```python
from build123d import *

# Parameters (mm, degrees)
ESQUISSE1_W             = 140
ESQUISSE1_H             = 40
ESQUISSE1_R             = 2.75
ESQUISSE1_R_2           = 1.6
ESQUISSE1_R_3           = 12.5
BOSS_EXTRU_1_DEPTH      = 2
ENL_V_MAT_EXTRU_1_REACH = 4
CONG_1_R                = 2


with BuildPart() as part:
    # Esquisse1 → Boss.-Extru.1 (new body)
    with BuildSketch(Plane(origin=(0, 0, 0), x_dir=(1, 0, 0), z_dir=(0, 1, 0))):
        Rectangle(ESQUISSE1_W, ESQUISSE1_H)
        with Locations((-61, 0)):
            Circle(ESQUISSE1_R, mode=Mode.SUBTRACT)
        with Locations((-29, 0)):
            Circle(ESQUISSE1_R, mode=Mode.SUBTRACT)
        with Locations((29, 0)):
            Circle(ESQUISSE1_R, mode=Mode.SUBTRACT)
        with Locations((61, 0)):
            Circle(ESQUISSE1_R, mode=Mode.SUBTRACT)
        with Locations((-15.5, 15.5)):
            Circle(ESQUISSE1_R_2, mode=Mode.SUBTRACT)
        with Locations((15.5, 15.5)):
            Circle(ESQUISSE1_R_2, mode=Mode.SUBTRACT)
        with Locations((15.5, -15.5)):
            Circle(ESQUISSE1_R_2, mode=Mode.SUBTRACT)
        with Locations((-15.5, -15.5)):
            Circle(ESQUISSE1_R_2, mode=Mode.SUBTRACT)
        Circle(ESQUISSE1_R_3, mode=Mode.SUBTRACT)
    extrude(amount=BOSS_EXTRU_1_DEPTH)

    # Esquisse2 → Enlèv. mat.-Extru.1 (cut, up to next)
    with BuildSketch(Plane.XZ, mode=Mode.PRIVATE) as enl_v_mat_extru_1_sk1:
        Polygon((22, -20), (22, -7.5), (67, -7.5), (67, 7.5), (22, 7.5), (22, 20), (70, 20), (70, -20), align=None)
    enl_v_mat_extru_1_tool1 = extrude(enl_v_mat_extru_1_sk1.sketch, amount=-ENL_V_MAT_EXTRU_1_REACH, mode=Mode.PRIVATE) & part.part
    add(enl_v_mat_extru_1_tool1.solids().sort_by_distance((22.62482, 0, -13.75))[0], mode=Mode.SUBTRACT)
    # Esquisse2 → Enlèv. mat.-Extru.1 (cut, up to next)
    with BuildSketch(Plane.XZ, mode=Mode.PRIVATE) as enl_v_mat_extru_1_sk2:
        Polygon((-70, 20), (-70, -20), (-22, -20), (-22, -7.5), (-67, -7.5), (-67, 7.5), (-22, 7.5), (-22, 20), align=None)
    enl_v_mat_extru_1_tool2 = extrude(enl_v_mat_extru_1_sk2.sketch, amount=-ENL_V_MAT_EXTRU_1_REACH, mode=Mode.PRIVATE) & part.part
    add(enl_v_mat_extru_1_tool2.solids().sort_by_distance((-69.37518, 0, 0))[0], mode=Mode.SUBTRACT)

    # Congé1
    cong_1_edges = [part.edges().sort_by_distance(p)[0] for p in [
        (22, 1, -7.5),
        (22, 1, 7.5),
        (-22, 1, 7.5),
        (-22, 1, -7.5),
    ]]
    fillet(cong_1_edges, radius=CONG_1_R)


solid = part.part
```
Can you work these out from the model? Positions are in its coordinate system, mm. Give positions to 0.01 mm unless a question says otherwise; leave off trailing zeros. Loops run counter-clockwise (first coordinate to the right, second up) from the corner with the lowest first, then second, coordinate; pieces in that order, holes last. Notation, with made-up numbers: M 11,8 L 47,8 A32 cw 47,40 Z; hole C 0,36.25 d2. An arc over 180 degrees is marked long. Answer in a Markdown table with one row per item.
1. For pin 1 Ø1 at (y, z) = (1, -17) entering from +X; pin 2 Ø1 at (x, y) = (-40.5, 1.5) entering from -Z; pin 3 Ø1 at (x, y) = (-44.5, 1) entering from +Z; pin 4 Ø5 at (x, z) = (-47, 11) entering from -Y, each with a flat end and sliding along its axis, tell me the tip position at first contact or that it passes through.
Taken from the geometry:
| item | result |
|---|---|
| pin 1 | stops at x = 22 |
| pin 2 | stops at z = -7.5 |
| pin 3 | stops at z = 7.5 |
| pin 4 | passes through |
2. Suppose I cut it at A-A on z = 0. Write out the boundary of the cut face in (x, y).
Taken from the geometry:
| item | result |
|---|---|
| outline | M -67,0 L -63.75,0 L -63.75,2 L -67,2 Z; M -58.25,0 L -31.75,0 L -31.75,2 L -58.25,2 Z; M -26.25,0 L -12.5,0 L -12.5,2 L -26.25,2 Z; M 12.5,0 L 26.25,0 L 26.25,2 L 12.5,2 Z; M 31.75,0 L 58.25,0 L 58.25,2 L 31.75,2 Z; M 63.75,0 L 67,0 L 67,2 L 63.75,2 Z |
3. Suppose I cut it at C-C on z = -15.5. Write out the boundary of the cut face in (x, y), plus the area to 3 significant figures.
Taken from the geometry:
| item | result |
|---|---|
| outline | M -22,0 L -17.1,0 L -17.1,2 L -22,2 Z; M -13.9,0 L 13.9,0 L 13.9,2 L -13.9,2 Z; M 17.1,0 L 22,0 L 22,2 L 17.1,2 Z |
| area | 75.2 mm² |
4. Thinking about a two-plate mould opening in Z: for faces 1 (the cylindrical face through (58.253, 0.986, -0.121)), 2 (the flat face through (-1, 2, -14)), which applies, released by +Z, released by -Z, zero draft, split by the parting line, or undercut?
Taken from the geometry:
| item | result |
|---|---|
| face 1 | undercut |
| face 2 | zero draft |
5. If I drill on line 1 along X through (y, z) = (0.8, 15.5); line 2 along X through (y, z) = (1.1, 0); line 3 along Z through (x, y) = (15.5, 1.15), over which ranges is the centre line in solid material (lowest first)?
Taken from the geometry:
| item | result |
|---|---|
| line 1 | x = -22 to -17.1, -13.9 to 13.9, 17.1 to 22 |
| line 2 | x = -67 to -63.75, -58.25 to -31.75, -26.25 to -12.5, 12.5 to 26.25, 31.75 to 58.25, 63.75 to 67 |
| line 3 | z = -20 to -17.1, -13.9 to 13.9, 17.1 to 20 |
6. Suppose I cut it at D-D on x = 15.5. Write out the boundary of the cut face in (y, z).
Taken from the geometry:
| item | result |
|---|---|
| outline | M 0,-20 L 2,-20 L 2,-17.1 L 0,-17.1 Z; M 0,-13.9 L 2,-13.9 L 2,13.9 L 0,13.9 Z; M 0,17.1 L 2,17.1 L 2,20 L 0,20 Z |
7. Suppose I cut it at B-B on x = -29. Write out the boundary of the cut face in (y, z).
Taken from the geometry:
| item | result |
|---|---|
| outline | M 0,-7.5 L 2,-7.5 L 2,-2.75 L 0,-2.75 Z; M 0,2.75 L 2,2.75 L 2,7.5 L 0,7.5 Z |
